from build123d import *

# Parameters (mm, degrees)
SKETCH_1_R      = 2.25
SKETCH_1_R_2    = 2
EXTRUDE_1_DEPTH = 2
SKETCH_2_W      = 10
SKETCH_2_H      = 6
EXTRUDE_2_DEPTH = 4
FILLET_1_R      = 2


with BuildPart() as part:
    # Эскиз1 → Бобышка-Вытянуть1 (new body)
    with BuildSketch(Plane(origin=(0, 0, 0), x_dir=(1, 0, 0), z_dir=(0, 1, 0))):
        Polygon((5, 31), (0, 18), (0, 0), (34, 0), (34, 18), (29, 31), align=None)
        with Locations(Location((6, 9, 0), (0, 0, 270))):
            Circle(SKETCH_1_R, mode=Mode.SUBTRACT)
        with Locations(Location((28, 9, 0), (0, 0, 270))):
            Circle(SKETCH_1_R, mode=Mode.SUBTRACT)
        with Locations(Location((12, 20, 0), (0, 0, 270))):
            Circle(SKETCH_1_R_2, mode=Mode.SUBTRACT)
        with Locations(Location((22, 20, 0), (0, 0, 270))):
            Circle(SKETCH_1_R_2, mode=Mode.SUBTRACT)
    extrude(amount=EXTRUDE_1_DEPTH)

    # Эскиз2 → Бобышка-Вытянуть2 (add)
    with BuildSketch(Plane(origin=(0, 2, 0), x_dir=(1, 0, 0), z_dir=(0, 1, 0))):
        with Locations((17, 9)):
            Rectangle(SKETCH_2_W, SKETCH_2_H)
    extrude(amount=EXTRUDE_2_DEPTH)

    # Скругление1
    fillet_1_edges = [part.edges().sort_by_distance(p)[0] for p in [
        (34, 1, -18),
        (34, 1, 0),
        (0, 1, 0),
        (0, 1, -18),
        (5, 1, -31),
        (29, 1, -31),
    ]]
    fillet(fillet_1_edges, radius=FILLET_1_R)


solid = part.part
Part model, mm, in its own coordinate system. A direction names the side the tool comes from. Coordinates: 2 decimals unless noted, no trailing zeros. Order: outer loops, then holes, each group sorted by start corner. A loop starts at its lowest first (then second) coordinate and runs counter-clockwise, first axis right, second up. Notation, with made-up numbers: M 84.5,2 L 133.5,2 A19 ccw 133.5,26 Z; hole C 30,-25.5 d8. An arc over 180 degrees is marked long. Use a Markdown table: item, result.
(1) Cut at A-A on z = -9. Write the cut outline in (x, y).
A:
| item | result |
|---|---|
| outline | M 0,0 L 3.75,0 L 3.75,2 L 0,2 Z; M 8.25,0 L 25.75,0 L 25.75,2 L 22,2 L 22,6 L 12,6 L 12,2 L 8.25,2 Z; M 30.25,0 L 34,0 L 34,2 L 30.25,2 Z |
(2) Pull direction Z, two halves, no side cores. Call faces 1 (the flat face through (17, 6, -9)), 2 (the flat face through (17, 1, -31)), 3 (the cylindrical face through (14, 1, -20)), 4 (the cylindrical face through (6.099, 0.986, -11.248)): released by +Z, released by -Z, zero draft, split by the parting line, or undercut.
A:
| item | result |
|---|---|
| face 1 | zero draft |
| face 2 | released by -Z |
| face 3 | undercut |
| face 4 | undercut |
(3) Cut at D-D on x = 6. Write the cut outline in (y, z).
A:
| item | result |
|---|---|
| outline | M 0,-30.96 L 2,-30.96 L 2,-11.25 L 0,-11.25 Z; M 0,-6.75 L 2,-6.75 L 2,0 L 0,0 Z |
(4) Flat gauge pins, fed straight in: pin 1 (2 mm diameter, centred on y = 4, z = -10.5, fed in from +X); pin 2 (1 mm diameter, centred on x = 5.5, y = 1, fed in from -Z); pin 3 (1.2 mm diameter, centred on x = 19.5, y = 3.5, fed in from +Z). Where does each tip first touch, or does it go through?
A:
| item | result |
|---|---|
| pin 1 | stops at x = 22 |
| pin 2 | stops at z = -30.96 |
| pin 3 | stops at z = -6 |
(5) Cut at B-B on y = 0.9. Write the cut outline in (x, z), then the cut area to 3 significant figures.
A:
| item | result |
|---|---|
| outline | M 0,-17.63 A2 ccw 0.13,-18.35 L 4.51,-29.72 A2 ccw 6.37,-31 L 27.63,-31 A2 ccw 29.49,-29.72 L 33.87,-18.35 A2 ccw 34,-17.63 L 34,-2 A2 ccw 32,0 L 2,0 A2 ccw 0,-2 Z; hole C 6,-9 d4.5; hole C 12,-20 d4; hole C 22,-20 d4; hole C 28,-9 d4.5 |
| area | 930 mm^2 |
(6) Probe L1, parallel to X at y = 1.5, z = -9; L2, parallel to X at y = 1.35, z = -20; L3, parallel to Y at x = 10.5, z = -29. List the from-to ranges inside material, lowest first.
A:
| item | result |
|---|---|
| L1 | x = 0 to 3.75, 8.25 to 25.75, 30.25 to 34 |
| L2 | x = 0.77 to 10, 14 to 20, 24 to 33.23 |
| L3 | y = 0 to 2 |
(7) Tool access for faces 5 (the flat face through (17, 4, -12)), 6 (the flat face through (12, 4, -9)), 7 (the flat face through (0, 1, -10)), 8 (the flat face through (17, 4, -6)), 9 (the flat face through (22, 4, -9)): list every direction of +Z, -Z, +X, -X, +Y, -Y with a clear straight run to the whole face (end or side of a thin tool).
A:
| item | result |
|---|---|
| face 5 | -Z, +X, -X, +Y |
| face 6 | +Z, -Z, -X, +Y |
| face 7 | +Z, -Z, -X, +Y, -Y |
| face 8 | +Z, +X, -X, +Y |
| face 9 | +Z, -Z, +X, +Y |
(8) Cut at C-C on x = 18.5. Write the cut outline in (y, z), then the cut area to 3 significant figures.
A:
| item | result |
|---|---|
| outline | M 0,-31 L 2,-31 L 2,-12 L 6,-12 L 6,-6 L 2,-6 L 2,0 L 0,0 Z |
| area | 86.0 mm^2 |
